Check sheet for the modelled part. Datum: model origin and axes. Units: mm. Face numbers are marked on the shaded views. A direction names the side the tool comes from. Round coordinates to 2 decimals unless told otherwise and drop trailing zeros. Loops run counter-clockwise (first coordinate to the right, second up) from the corner with the lowest first, then second, coordinate; pieces in that order, holes last. Notation, with made-up numbers: M 68.5,83 L 84.5,83 A23 ccw 84.5,113 Z; hole C 10,69 d9. An arc over 180 degrees is marked long. Write item = value, one per line. Start each with the question number.
(1) Set-up check for the marked faces 4 and 5: record each of +Z, -Z, +X, -X, +Y, -Y from which the full face is reachable in a straight line by a thin tool's end or side.
(2) Cross-section at C-C on y = -50. Record the boundary of the cut face in (x, z), plus the area to 3 significant figures.
(3) Mould release check, pull along Y, two halves, no side actions. Record for the marked faces 1, 2 and 3: pulls with the +Y half, pulls with the -Y half, needs draft (parallel to the pull), parting line crosses it, or undercut.
(4) Go/stop test with flat-tipped pins: P1, Ø2, axis at x = 60, y = -50, coming from the -Z side; P2, Ø3.5, axis at x = 100, y = -50, coming from the -Z side. Record where each tip stops, or that it passes through.
(5) Cross-section at B-B on x = 100. Record the boundary of the cut face in (y, z), plus the area to 3 significant figures.
(6) Scan lines: L1, parallel to Y at x = 100, z = 9.85; L2, parallel to Y at x = 100, z = 6; L3, parallel to X at y = -55, z = 4. Record each from-to range of solid material in increasing order. Write a range as from..to.
(7) Cross-section at D-D on y = -44.75. Record the boundary of the cut face in (x, z).
(8) Cross-section at A-A on z = 12.25. Record the boundary of the cut face in (x, y), plus the area to 3 significant figures.
from build123d import *

# Parameters (mm, degrees)
SKETCH003_W     = 50
SKETCH003_H     = 20
PAD001_DEPTH    = 14
SKETCH004_R     = 13.5
POCKET002_DEPTH = 20.001
SKETCH005_R     = 1.3
POCKET003_DEPTH = 14.001
SKETCH017_R     = 3
POCKET012_DEPTH = 8


with BuildPart() as part:
    # Sketch003 → Pad001 (new body)
    with BuildSketch(Plane.XY):
        Rectangle(SKETCH003_W, SKETCH003_H)
    extrude(amount=PAD001_DEPTH)

    # Sketch004 (on Face3 of Pad001) → Pocket002 (cut, through all)
    with BuildSketch(Plane.XZ.offset(10)):
        with Locations((0, 15)):
            Circle(SKETCH004_R)
    extrude(amount=-POCKET002_DEPTH, mode=Mode.SUBTRACT)

    # Sketch005 (on Face6 of Pocket002) → Pocket003 (cut, through all)
    with BuildSketch(Plane.XY.offset(14)):
        with Locations((-20, 0)):
            Circle(SKETCH005_R)
        with Locations((20, 0)):
            Circle(SKETCH005_R)
    extrude(amount=-POCKET003_DEPTH, mode=Mode.SUBTRACT)

    # Sketch017 (on Face2 of Pocket003) → Pocket012 (cut)
    with BuildSketch(Plane(origin=(0, 0, 0), x_dir=(1, 0, 0), z_dir=(0, 0, -1))):
        with Locations((-20, 0)):
            Circle(SKETCH017_R)
        with Locations((20, 0)):
            Circle(SKETCH017_R)
    extrude(amount=-POCKET012_DEPTH, mode=Mode.SUBTRACT)


with BuildPart() as part_1:
    # Body001 placement: moved
    add(part.part.moved(Location((80, -50, 0))))


solid = part_1.part
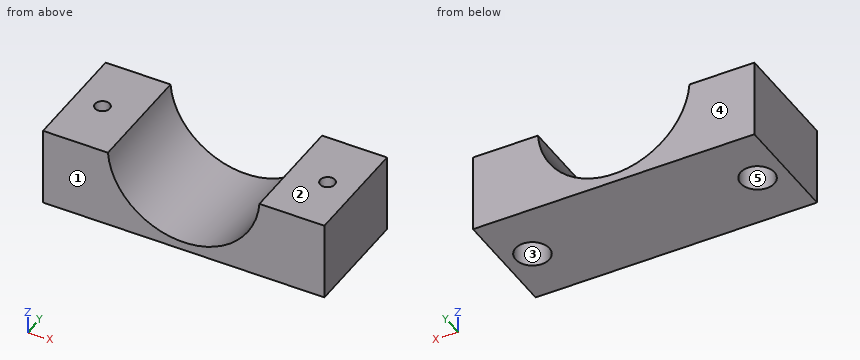
Result:
q1.face_4 = +Z, -Z, +X, -X, +Y
q1.face_5 = -Z
q2.outline = M 55,0 L 57,0 L 57,8 L 58.7,8 L 58.7,14 L 55,14 Z; M 61.3,8 L 63,8 L 63,0 L 97,0 L 97,8 L 98.7,8 L 98.7,14 L 93.46,14 A13.5 cw 66.54,14 L 61.3,14 Z; M 101.3,8 L 103,8 L 103,0 L 105,0 L 105,14 L 101.3,14 Z
q2.area = 313 mm^2
q3.face_1 = pulls with the -Y half
q3.face_2 = needs draft
q3.face_3 = undercut
q4.P1 = through
q4.P2 = 8
q5.outline = M -60,0 L -53,0 L -53,8 L -51.3,8 L -51.3,14 L -60,14 Z; M -48.7,8 L -47,8 L -47,0 L -40,0 L -40,14 L -48.7,14 Z
q5.area = 216 mm^2
q6.L1 = -60..-51.3, -48.7..-40
q6.L2 = -60..-53, -47..-40
q6.L3 = 55..72.17, 87.83..105
q7.outline = M 55,0 L 105,0 L 105,14 L 93.46,14 A13.5 cw 66.54,14 L 55,14 Z
q8.outline = M 55,-60 L 66.78,-60 L 66.78,-40 L 55,-40 Z; M 93.22,-60 L 105,-60 L 105,-40 L 93.22,-40 Z; hole C 60,-50 d2.6; hole C 100,-50 d2.6
q8.area = 461 mm^2
